Source: CAD feature listing. Evaluate the final solid. Frame: model axes, mm. Round coordinates to 2 decimals unless told otherwise and drop trailing zeros. Loops run counter-clockwise (first coordinate to the right, second up) from the corner with the lowest first, then second, coordinate; pieces in that order, holes last.
Item 1: Pull-direction query (X, two-part tool) for faces 1 (the cylindrical face through (-16.213, 1.972, -53.196)), 2 (the flat face through (0, 4, -31)), 3 (the cylindrical face through (-2.8, 2.03, -26.93)), 4 (the cylindrical face through (-11.43, 1.97, -74.01)); classes: released by +X, released by -X, zero draft, split by the parting line, or undercut.
Item 2: Ray query, L1, parallel to Z at x = 11, y = 3.2; L2, parallel to X at y = 2.4, z = -100.74; L3, parallel to Z at x = -4.5, y = 2.5. Return the intervals inside material, ascending.
Item 3: First-contact query: P1, Ø1.5, axis at y = 1.5, z = -67, coming from the -X side; P2, Ø1, axis at x = 17.5, y = 0.5, coming from the -Z side (3 decimals); P3, Ø1, axis at x = -8, y = 1.5, coming from the +Z side. Flat tips, straight axial feed; report the tip coordinate or a pass-through.
Item 4: Section query B-B on x = -11.5. Return loops of the section in (y, z), then the cut area to 3 significant figures.
Item 5: Section query D-D on z = -55.74. Return loops of the section in (x, y), then the cut area to 3 significant figures.
Item 6: Section query C-C on y = 3.25. Give the number of separate pieces and of enclosed holes in the cut face, then the cut area to 3 significant figures.
Item 7: Section query A-A on z = -100.74. Return loops of the section in (x, y), then the cut area to 3 significant figures.
```python
from build123d import *

# Parameters (mm, degrees)
EXTRUDE_1_DEPTH          = 4
SKETCH_2_R               = 2.1
CUT_EXTRUDE_1_DEPTH      = 4
PATTERN_CIRCULAR_1_COUNT = 3
SKETCH_4_R               = 7.5
CUT_EXTRUDE_2_DEPTH      = 27.5
SKETCH_5_R               = 1.65
CUT_EXTRUDE_3_DEPTH      = 27.5
PATTERN_CIRCULAR_2_COUNT = 3
SKETCH_6_R               = 15
CUT_EXTRUDE_4_DEPTH      = 29.5


with BuildPart() as part:
    # 草图1 → 凸台-拉伸1 (new body)
    with BuildSketch(Plane(origin=(0, 0, 0), x_dir=(1, 0, 0), z_dir=(0, 1, 0))):
        with BuildLine():
            ThreePointArc((26.78524518, 13.511130252), (16.244949948, 52.625392683), (22.086079359, 92.711606726))
            ThreePointArc((22.086079359, 92.711606726), (0, 124.24), (-22.086079359, 92.711606726))
            ThreePointArc((-22.086079359, 92.711606726), (-16.244949948, 52.625392683), (-26.78524518, 13.511130252))
            ThreePointArc((-26.78524518, 13.511130252), (0, -30), (26.78524518, 13.511130252))
        make_face()
    extrude(amount=EXTRUDE_1_DEPTH)

    # 草图2 → 切除-拉伸1 (cut)
    with BuildSketch(Plane(origin=(0, 4, 0), x_dir=(1, 0, 0), z_dir=(0, 1, 0))):
        with Locations(Location((22.952521328, -9.908671188, 0), (0, 0, 270))):
            Circle(SKETCH_2_R)
    cut_extrude_1 = extrude(amount=-CUT_EXTRUDE_1_DEPTH, mode=Mode.SUBTRACT)

    # 阵列(圆周)1: 切除-拉伸1 ×3 about axis
    pattern_circular_1_axis = Axis((0, 0, 0), (0, 1, 0))
    for i in range(1, PATTERN_CIRCULAR_1_COUNT):
        add(cut_extrude_1.rotate(pattern_circular_1_axis, i * 360 / PATTERN_CIRCULAR_1_COUNT), mode=Mode.SUBTRACT)

    # 草图4 → 切除-拉伸2 (cut)
    with BuildSketch(Plane(origin=(0, 0, 0), x_dir=(-1, 0, 0), z_dir=(0, -1, 0))):
        with Locations(Location((0, 55.74, 0), (0, 0, 90))):
            Circle(SKETCH_4_R)
    extrude(amount=-CUT_EXTRUDE_2_DEPTH, mode=Mode.SUBTRACT)

    # 草图5 → 切除-拉伸3 (cut)
    with BuildSketch(Plane.XZ):
        with Locations(Location((-11.5, -35.821415713, 0), (0, 0, 270))):
            Circle(SKETCH_5_R)
        with Locations(Location((11.5, -35.821415713, 0), (0, 0, 270))):
            Circle(SKETCH_5_R)
    cut_extrude_3 = extrude(amount=-CUT_EXTRUDE_3_DEPTH, mode=Mode.SUBTRACT)

    # 阵列(圆周)2: 切除-拉伸3 ×3 about axis
    pattern_circular_2_axis = Axis((0, 0, -55.74), (0, 1, 0))
    for i in range(1, PATTERN_CIRCULAR_2_COUNT):
        add(cut_extrude_3.rotate(pattern_circular_2_axis, i * 360 / PATTERN_CIRCULAR_2_COUNT), mode=Mode.SUBTRACT)

    # 草图6 → 切除-拉伸4 (cut)
    with BuildSketch(Plane.XZ):
        with Locations(Location((0, -100.74, 0), (0, 0, 270))):
            Circle(SKETCH_6_R)
    extrude(amount=-CUT_EXTRUDE_4_DEPTH, mode=Mode.SUBTRACT)


solid = part.part
```
Data:
1. face 1: released by -X
1. face 2: zero draft
1. face 3: undercut
1. face 4: undercut
2. L1: z = -121.51 to -110.94, -90.54 to -77.23, -74.09 to -37.39, -34.25 to 27.91
2. L2: x = -23.5 to -15, 15 to 23.5
2. L3: z = -123.81 to -115.05, -86.43 to -61.74, -49.74 to -26.19, -23.48 to 29.66
3. P1: stops at x = -16.49
3. P2: stops at z = -116.965
3. P3: stops at z = 29.05
4. outline: (0, -121.23) - (4, -121.23) - (4, -110.37) - (0, -110.37) - close; (0, -91.11) - (4, -91.11) - (4, -77.31) - (0, -77.31) - close; (0, -74.01) - (4, -74.01) - (4, -37.47) - (0, -37.47) - close; (0, -34.17) - (4, -34.17) - (4, 27.71) - (0, 27.71) - close
4. area: 492 mm2
5. outline: (-16.11, 0) - (-7.5, 0) - (-7.5, 4) - (-16.11, 4) - close; (7.5, 0) - (16.11, 0) - (16.11, 4) - (7.5, 4) - close
5. area: 68.9 mm2
6. separate pieces: 1
6. enclosed holes: 9
6. area: 5,470 mm2
7. outline: (-23.5, 0) - (-15, 0) - (-15, 4) - (-23.5, 4) - close; (15, 0) - (23.5, 0) - (23.5, 4) - (15, 4) - close
7. area: 68.0 mm2
